Autodesk Fusion 360 part; units mm, degrees
sketch "Sketch1" plane through (0, 0, 0) normal (0, 1, 0) x (1, 0, 0)
  line L0 (0, 3.2328) -> (70, 3.2328)
  line L1 (70, 3.2328) -> (70, -51.7672)
  line L2 (70, -51.7672) -> (0, -51.7672)
  line L3 (0, -51.7672) -> (0, 3.2328)
  dimension "d1" = 70
  dimension "d2" = 55
  dimension "d3" = 55
extrude "Extrude1" add sketch "Sketch1" along normal mid plane 30
sketch "Sketch2" plane through (70, 0, 0) normal (1, 0, 0) x (0, 0, -1)
  line L0 (3.2328, -15) -> (3.2328, 15)
  line L1 (3.2328, 15) -> (-51.7672, 15)
  line L2 (-51.7672, 15) -> (-51.7672, -15)
  line L3 (-51.7672, -15) -> (3.2328, -15)
  line L4 (-6.7672, -15) -> (-6.7672, -7)
  line L5 (-6.7672, -7) -> (-51.7672, -7)
  dimension "d6" = 10
  dimension "d7" = 45
  dimension "d8" = 8
extrude "Extrude2" cut sketch "Sketch2" against normal blind 90 contours L2 L3 L4 L5
sketch "Sketch3" plane through (0, 15, 0) normal (0, 1, 0) x (-1, 0, 0)
  line L0 (0, 51.7672) -> (-70, 51.7672)
  line L1 (-70, 51.7672) -> (-70, -3.2328)
  line L2 (-70, -3.2328) -> (0, -3.2328)
  line L3 (0, -3.2328) -> (0, 51.7672)
  circle A0 centre (-18, 21.7672) radius 11
  circle A1 centre (-52, 21.7672) radius 11
  dimension "d11" = 22
  dimension "d12" = 22
  dimension "d13" = 30
  dimension "d14" = 18
  dimension "d15" = 34
extrude "Extrude3" cut sketch "Sketch3" against normal blind 50 contours A0 | A1
sketch "Sketch4" plane through (0, 15, 0) normal (0, 1, 0) x (-1, 0, 0)
  circle A0 centre (-52, 21.7672) radius 11
  circle A1 centre (-18, 21.7672) radius 11
  line L0 (0, 51.7672) -> (-70, 51.7672)
  line L1 (-70, 51.7672) -> (-70, -3.2328)
  line L2 (-70, -3.2328) -> (0, -3.2328)
  line L3 (0, -3.2328) -> (0, 51.7672)
  line L4 (-45, 51.7672) -> (-45, 101.7672)
  line L5 (-45, 101.7672) -> (-70, 101.7672)
  line L6 (-70, 101.7672) -> (-70, 51.7672)
  dimension "d18" = 50
  dimension "d19" = 50
  dimension "d20" = 25
extrude "Extrude4" add sketch "Sketch4" against normal blind 17 contours L0 L4 L5 L6
sketch "Sketch5" plane through (70, 0, 0) normal (1, 0, 0) x (0, 0, -1)
  line L0 (-51.7672, -7) -> (-6.7672, -7)
  line L1 (-6.7672, -7) -> (-6.7672, -15)
  line L2 (-6.7672, -15) -> (3.2328, -15)
  line L3 (3.2328, -15) -> (3.2328, 15)
  line L4 (3.2328, 15) -> (-101.7672, 15)
  line L5 (-101.7672, 15) -> (-101.7672, -2)
  line L6 (-101.7672, -2) -> (-51.7672, -2)
  line L7 (-51.7672, -2) -> (-51.7672, -7)
  line L8 (-170, 80) -> (-115.9179, 80)
  line L9 (-170, 60) -> (-114.0006, 60)
  line L10 (-116.7673, 45) -> (-116.7673, 13)
  arc A0 (-116.7673, 13) -> (-101.7672, -2) centre (-101.7673, 13) ccw
  line L11 (-116.7673, 45) -> (-102.1531, 45)
  line L12 (-102.1531, 45) -> (-101.7672, 15)
  dimension "d25" = 32
  dimension "d26" = 15
  dimension "d27" = 30
extrude "Extrude5" add sketch "Sketch5" against normal blind 25 contours L5 L10 A0 L11 L12
sketch "Sketch6" plane through (0, 0, 116.7673) normal (0, 0, 1) x (1, 0, 0)
  line L0 (70, 13) -> (70, 45)
  line L1 (70, 45) -> (45, 45)
  line L2 (45, 45) -> (45, 13)
  line L3 (45, 13) -> (70, 13)
  line L4 (45, 45) -> (34.5, 45)
  line L5 (34.5, 45) -> (34.5, 70)
  line L6 (34.5, 70) -> (42.5, 70)
  line L7 (42.5, 70) -> (42.5, 60)
  line L8 (42.5, 60) -> (72.5, 60)
  line L9 (72.5, 60) -> (72.5, 70)
  line L10 (72.5, 70) -> (80.5, 70)
  line L11 (80.5, 70) -> (80.5, 45)
  line L12 (80.5, 45) -> (70, 45)
  dimension "d30" = 25
  dimension "d31" = 8
  dimension "d32" = 8
  dimension "d33" = 25
  dimension "d34" = 10.5
  dimension "d35" = 10.5
  dimension "d36" = 30
  dimension "d37" = 46
extrude "Extrude6" add sketch "Sketch6" along normal blind 25 and the other way blind 15 contours L1 L4 L5 L6 L7 L8 L9 L10 L11 L12
Source: CAD feature listing. Evaluate the final solid. Frame: model axes, mm. A direction names the side the tool comes from. Coordinates: 2 decimals unless noted, no trailing zeros. Write each loop counter-clockwise with the first axis right and the second up, starting at its lowest first coordinate (ties: lowest second). Pieces come first, ordered by that corner, then holes. Notation, with made-up numbers: (-13, -14.75) - (32, -14.75) arc R28 ccw to (32, 21.25) - close; hole circle Ø11 at (37.25, -24.75). An arc over 180 degrees is marked (long way). Answer as a JSON object with one key per item and string values.
Q1. Section query B-B, the plane z = 30. Output: boundary loops of the cut face in (x, y), plus the area to 3 significant figures.
Ans:
{"outline": "(0, -7) - (10.7, -7) - (10.7, 15) - (0, 15) - close; (25.3, -7) - (44.7, -7) - (44.7, 15) - (25.3, 15) - close; (59.3, -7) - (70, -7) - (70, 15) - (59.3, 15) - close", "area": "898 mm2"}
Q2. Draft query along X for faces 1 (the cylindrical face through (54.385, 4.154, 11.029)), 2 (the flat face through (0, 3, 25)), 3 (the flat face through (35, -15, 2)). Return one class per face: released by +X, released by -X, zero draft, split by the parting line, or undercut.
Ans:
{"face 1": "undercut", "face 2": "released by -X", "face 3": "zero draft"}
Q3. Section query C-C, the plane y = 56.5. Output: boundary loops of the cut face in (x, z).
Ans:
{"outline": "(34.5, 101.77) - (80.5, 101.77) - (80.5, 141.77) - (34.5, 141.77) - close"}
Q4. Section query A-A, the plane x = 18. Output: boundary loops of the cut face in (y, z), plus the area to 3 significant figures.
Ans:
{"outline": "(-15, -3.23) - (15, -3.23) - (15, 10.77) - (-7, 10.77) - (-7, 6.77) - (-15, 6.77) - close; (-7, 32.77) - (15, 32.77) - (15, 51.77) - (-7, 51.77) - close", "area": "806 mm2"}
Q5. Section query D-D, the plane z = 132. Output: boundary loops of the cut face in (x, y).
Ans:
{"outline": "(34.5, 45) - (80.5, 45) - (80.5, 70) - (72.5, 70) - (72.5, 60) - (42.5, 60) - (42.5, 70) - (34.5, 70) - close"}
Q6. First-contact query: pin 1 Ø7.5 at (y, z) = (52, 115.5) entering from -X; pin 2 Ø15 at (x, z) = (53, 118.5) entering from +Y; pin 3 Ø4 at (x, z) = (70, 98) entering from -Y. Flat tips, straight axial feed; report the tip coordinate or a pass-through.
Ans:
{"pin 1": "stops at x = 34.5", "pin 2": "stops at y = 60", "pin 3": "stops at y = -2"}
Q7. Set-up query: faces 4 (the flat face through (57, 60, 121)), 5 (the flat face through (70, 11, 61)), 6 (the flat face through (43, 15, 38)), 7 (the flat face through (35, -11, 6.767)). Return all of +Z, -Z, +X, -X, +Y, -Y with unobstructed straight access to the full face (end or side cutting, diameter ignored); none if empty.
Ans:
{"face 4": "+Z, -Z, +Y", "face 5": "+Z, -Z, +X, -Y", "face 6": "-Z, +X, -X, +Y", "face 7": "+Z, +X, -X, -Y"}
Q8. Material intervals for line 1 (Y direction, x = 34.5, z = 5.5); line 2 (Y direction, x = 40.5, z = 121); line 3 (Z direction, x = 18, y = 2), sorted ascending. Write a range as [from, to].
Ans:
{"line 1": "y = [-15, 15]", "line 2": "y = [45, 70]", "line 3": "z = [-3.23, 10.77], [32.77, 51.77]"}
